```python
from build123d import *

# Parameters (mm, degrees)
SKETCH2_R                                      = 1.5875
SKETCH2_R_2                                    = 4.05
BOSS_EXTRUDE1_DEPTH                            = 3.175
CSK_FOR_6_FLAT_HEAD_MACHINE_SCREW1_D           = 3.6576
CSK_FOR_6_FLAT_HEAD_MACHINE_SCREW1_DEPTH       = 10.973
CSK_FOR_6_FLAT_HEAD_MACHINE_SCREW1_CSINK_D     = 7.0866
CSK_FOR_6_FLAT_HEAD_MACHINE_SCREW1_CSINK_ANGLE = 82
CSK_FOR_6_FLAT_HEAD_MACHINE_SCREW1_TIP         = 1.0988539
FILLET1_R                                      = 10


with BuildPart() as part:
    # Sketch2 → Boss-Extrude1 (new body)
    with BuildSketch(Plane.XY):
        with BuildLine():
            Line((8.170067778, -35.040125463), (-35.040125463, 8.170067778))
            ThreePointArc((-35.040125463, 8.170067778), (-34.032148119, 11.677897689), (-32.673983585, 15.065563272))
            Line((-32.673983585, 15.065563272), (-5.448690981, 74.111398302))
            ThreePointArc((-5.448690981, 74.111398302), (1.286050954, 77.459627628), (6, 71.599075355))
            Line((6, 71.599075355), (6, 20.870057685))
            Line((6, 20.870057685), (35.040125463, -8.170067778))
            ThreePointArc((35.040125463, -8.170067778), (25.441701987, -25.441701987), (8.170067778, -35.040125463))
        make_face()
        with Locations((0, 71.599075355)):
            Circle(SKETCH2_R, mode=Mode.SUBTRACT)
        with Locations((0, 65.599075355)):
            Circle(SKETCH2_R, mode=Mode.SUBTRACT)
        Circle(SKETCH2_R_2, mode=Mode.SUBTRACT)
    extrude(amount=-BOSS_EXTRUDE1_DEPTH)

    # CSK for #6 Flat Head Machine Screw1
    with Locations(Plane(origin=(0, 0, -3.175), x_dir=(-1, 0, 0), z_dir=(0, 0, -1))):
        with Locations((-7.071067812, 12.727922061), (-27.577164466, -7.778174593), (10.886616003, -8.91237387), (-7.778174593, -27.577164466)):
            CounterSinkHole(CSK_FOR_6_FLAT_HEAD_MACHINE_SCREW1_D / 2, CSK_FOR_6_FLAT_HEAD_MACHINE_SCREW1_CSINK_D / 2, depth=CSK_FOR_6_FLAT_HEAD_MACHINE_SCREW1_DEPTH, counter_sink_angle=CSK_FOR_6_FLAT_HEAD_MACHINE_SCREW1_CSINK_ANGLE)
            with Locations((0, 0, -(CSK_FOR_6_FLAT_HEAD_MACHINE_SCREW1_DEPTH + CSK_FOR_6_FLAT_HEAD_MACHINE_SCREW1_TIP / 2))):  # 118° drill point
                Cone(0, CSK_FOR_6_FLAT_HEAD_MACHINE_SCREW1_D / 2, CSK_FOR_6_FLAT_HEAD_MACHINE_SCREW1_TIP, mode=Mode.SUBTRACT)

    # Fillet1
    fillet1_edges = [part.edges().sort_by_distance(p)[0] for p in [
        (-35.040125463, 8.170067778, -1.5875),
    ]]
    fillet(fillet1_edges, radius=FILLET1_R)


solid = part.part
```
The model under review builds one solid part; all positions refer to its coordinate system, in mm. Coordinates: 2 decimals unless noted, no trailing zeros. Write each loop counter-clockwise with the first axis right and the second up, starting at its lowest first coordinate (ties: lowest second). Pieces come first, ordered by that corner, then holes. Notation, with made-up numbers: (-13, 44) - (23, 44) arc R21 cw to (23, 82) - close; hole circle Ø6 at (72.25, 55). An arc over 180 degrees is marked (long way). Answer in a Markdown table with one row per item. Add a question column.
Q1. Consider section A-A on y = 0. Give the boundary of the cut face in (x, z) (3 decimals).
Q2. Consider section D-D on y = -15. Give the boundary of the cut face in (x, z) (3 decimals).
Q3. To check wall thickness, follow line 1 along Y through (x, z) = (0, -0.8); line 2 along Y through (x, z) = (8, -2.6); line 3 along X through (y, z) = (-9, -2.6). State the ranges of each line that lie inside material, in increasing order. Write a range as from..to.
Q4. Consider section C-C on x = 0. Give the boundary of the cut face in (y, z) (3 decimals).
Q5. Draft analysis for pull direction X (two halves, no side actions). For faces 1 (the face through (1, 10, 0)), 2 (the face through (6, 47, -2)), 3 (the face through (-0.207, 67.173, -1.565)), state which applies: +X half, -X half, draft (parallel to the pull), parting line (faces both ways), or undercut.
Q6. Clearance check with flat-ended pins moving along their axes: pin 1 (1.6 mm diameter, centred on y = 58, z = -1, fed in from +X); pin 2 (6 mm diameter, centred on x = 7.07, y = 12.73, fed in from -Z); pin 3 (8 mm diameter, centred on x = 6, y = 45, fed in from +Z). State where each tip first meets the part, or that it passes through.
Q7. Consider section B-B on z = -1.7. Give the number of separate pieces and of enclosed holes in the cut face, then the cut area to 3 significant figures.
Answers below:
| question | item | result |
|---|---|---|
| 1 | outline | (-26.87, -3.175) - (-4.05, -3.175) - (-4.05, 0) - (-26.87, 0) - close; (4.05, -3.175) - (26.87, -3.175) - (26.87, 0) - (4.05, 0) - close |
| 2 | outline | (-11.87, -3.175) - (32.704, -3.175) - (32.704, 0) - (-11.87, 0) - close |
| 3 | line 1 | -26.87..-4.05, 4.05..64.01, 67.19..70.01, 73.19..77.6 |
| 3 | line 2 | -34.87..-30.61, -24.54..9.83, 15.63..18.87 |
| 3 | line 3 | -17.87..-13.93, -7.84..24.79, 30.36..34.84 |
| 4 | outline | (-26.87, -3.175) - (-4.05, -3.175) - (-4.05, 0) - (-26.87, 0) - close; (4.05, -3.175) - (64.012, -3.175) - (64.012, 0) - (4.05, 0) - close; (67.187, -3.175) - (70.012, -3.175) - (70.012, 0) - (67.187, 0) - close; (73.187, -3.175) - (77.599, -3.175) - (77.599, 0) - (73.187, 0) - close |
| 5 | face 1 | draft |
| 5 | face 2 | +X half |
| 5 | face 3 | undercut |
| 6 | pin 1 | x = 6 |
| 6 | pin 2 | z = -2.55 |
| 6 | pin 3 | z = 0 |
| 7 | separate pieces | 1 |
| 7 | enclosed holes | 7 |
| 7 | area | 3,460 mm² |
